```python
from build123d import *

# Parameters (mm, degrees)
F0_W      = 551
F0_H      = 330
F0_W_2    = 543
F0_H_2    = 320
F1_DEPTH  = 180
F3_DEPTH  = 551.001
F4_W      = 10
F4_H      = 30
F5_DEPTH  = 551
F6_W      = 5
F6_H      = 30
F7_DEPTH  = 160
F8_W      = 5
F8_H      = 30
F9_DEPTH  = 160
F10_R     = 10
F11_DEPTH = 25
F12_DEPTH = 170.001
F13_R     = 10
F14_DEPTH = 25


with BuildPart() as f1:
    # F0 (on Front) → F1 (new body)
    with BuildSketch(Plane.XZ):
        with Locations((275.5, 165)):
            Rectangle(F0_W, F0_H)
        with Locations((275.5, 165)):
            Rectangle(F0_W_2, F0_H_2, mode=Mode.SUBTRACT)
    extrude(amount=F1_DEPTH)

    # F2 (on face) → F3 (cut, through all)
    with BuildSketch(Plane.YZ.offset(551)):
        with BuildLine():
            Line((-180, 120), (-180, 210))
            ThreePointArc((-180, 210), (-225, 165), (-180, 120))
        make_face()
        with BuildLine():
            ThreePointArc((-180, 120), (-148.180195, 133.180195), (-135, 165))
            ThreePointArc((-135, 165), (-148.180195, 196.819805), (-180, 210))
            Line((-180, 210), (-180, 120))
        make_face()
    extrude(amount=-F3_DEPTH, mode=Mode.SUBTRACT)

    # F4 (on face) → F5 (join, through all)
    with BuildSketch(Plane.YZ.offset(551)):
        with Locations((-175, -15)):
            Rectangle(F4_W, F4_H)
        with Locations((-5, -15)):
            Rectangle(F4_W, F4_H)
        with Locations((-175, 345)):
            Rectangle(F4_W, F4_H)
        with Locations((-5, 345)):
            Rectangle(F4_W, F4_H)
    extrude(amount=-F5_DEPTH)

    # F6 (on face) → F7 (join, through all)
    with BuildSketch(Plane.XZ.offset(10)):
        with Locations((110.6, -15)):
            Rectangle(F6_W, F6_H)
        with Locations((221.2, -15)):
            Rectangle(F6_W, F6_H)
        with Locations((331.8, -15)):
            Rectangle(F6_W, F6_H)
        with Locations((442.4, -15)):
            Rectangle(F6_W, F6_H)
    extrude(amount=F7_DEPTH)

    # F8 (on face) → F9 (join, through all)
    with BuildSketch(Plane.XZ.offset(10)):
        with Locations((440.4, 345)):
            Rectangle(F8_W, F8_H)
        with Locations((329.8, 345)):
            Rectangle(F8_W, F8_H)
        with Locations((219.2, 345)):
            Rectangle(F8_W, F8_H)
        with Locations((108.6, 345)):
            Rectangle(F8_W, F8_H)
    extrude(amount=F9_DEPTH)

    # F10 (on face) → F11 (cut)
    with BuildSketch(Plane(origin=(0, -170, 0), x_dir=(-1, 0, 0), z_dir=(0, 1, 0))):
        with Locations((-165.959219, -12.5)):
            Circle(F10_R)
        with Locations((-387.1, -12.5)):
            Circle(F10_R)
        with Locations((-163.9, 345)):
            Circle(F10_R)
        with Locations((-385.1, 342.5)):
            Circle(F10_R)
    extrude(amount=-F11_DEPTH, mode=Mode.SUBTRACT)

    # F10 (on face) → F12 (cut, through all)
    with BuildSketch(Plane(origin=(0, -170, 0), x_dir=(-1, 0, 0), z_dir=(0, 1, 0))):
        with Locations((-163.9, 345)):
            Circle(F10_R)
        with Locations((-385.1, 342.5)):
            Circle(F10_R)
        with Locations((-165.959219, -12.5)):
            Circle(F10_R)
        with Locations((-387.1, -12.5)):
            Circle(F10_R)
    extrude(amount=F12_DEPTH, mode=Mode.SUBTRACT)

    # F13 (on face) → F14 (cut)
    with BuildSketch(Plane.XZ.offset(180)):
        with Locations((274.5, 342.5)):
            Circle(F13_R)
        with Locations((276.5, -12.5)):
            Circle(F13_R)
    extrude(amount=-F14_DEPTH, mode=Mode.SUBTRACT)


solid = f1.part
```
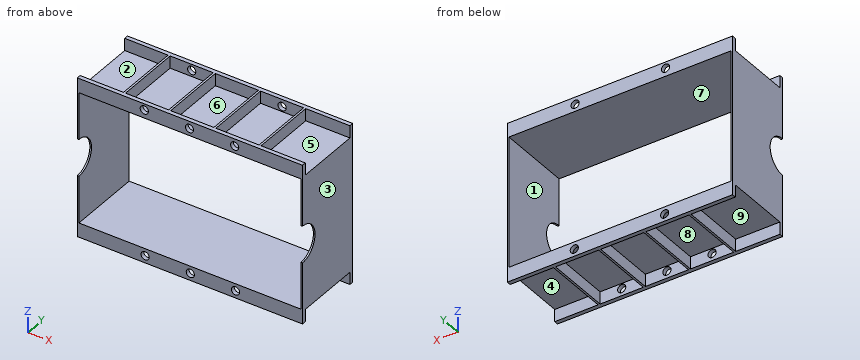
CAD build for the part. Positions are in the model's coordinates, mm. Face numbers are marked on the shaded views. A direction names the side the tool comes from. Coordinates: 2 decimals unless noted, no trailing zeros. Write each loop counter-clockwise with the first axis right and the second up, starting at its lowest first coordinate (ties: lowest second). Pieces come first, ordered by that corner, then holes. Notation, with made-up numbers: (-4.5, 57) -> (32.5, 57) arc R29 cw to (32.5, 92) -> close; hole circle Ø8 at (34.5, 81). An arc over 180 degrees is marked (long way). Return JSON: item names as keys, results as strings. Group by question number.
Q1. Pull direction Z, two halves, no side cores. Call the marked faces 1, 2, 3 and 4: released by +Z, released by -Z, zero draft, split by the parting line, or undercut.
Q2. Flat gauge pins, fed straight in: pin 1 (10 mm diameter, centred on x = 170.5, y = -144, fed in from -Z); pin 2 (3 mm diameter, centred on y = -66.5, z = 288, fed in from -X); pin 3 (2 mm diameter, centred on x = 163.5, y = -130, fed in from +Z); pin 4 (9 mm diameter, centred on y = -76.5, z = -9, fed in from -X). Where does each tip first touch, or does it go through?
Q3. Which spindle directions (+Z, -Z, +X, -X, +Y, -Y) get a long thin tool onto all of the face, cutting with end or side? Do the marked faces 5, 6, 7, 8 and 9. Say none if no direction does.
Q4. Drill centre lines: line 1 (X direction, y = -7.5, z = -12.5); line 2 (Z direction, x = 276, y = -176); line 3 (Z direction, x = 521, y = -143). Where is each one in solid material? Low to high.
Q5. Cut at C-C, the plane x = 163.9. State how many separate pieces and enclosed holes the cut face has, then the cut area to 3 significant figures.
Q6. Cut at B-B, the plane z = 232.5. Give the cut face in (x, y).
Q7. Cut at A-A, the plane x = 301.5. Give the cut face in (y, z), then the cut area to 3 significant figures.
Returned:
{
 "1": {"face 1": "undercut", "face 2": "released by +Z", "face 3": "zero draft", "face 4": "released by -Z"},
 "2": {"pin 1": "stops at z = 0", "pin 2": "stops at x = 0", "pin 3": "stops at z = 330", "pin 4": "stops at x = 108.1"},
 "3": {"face 5": "+Z, +X", "face 6": "+Z", "face 7": "+Y, -Y", "face 8": "-Z", "face 9": "-Z, -X"},
 "4": {"line 1": "x = 0 to 155.96, 175.96 to 377.1, 397.1 to 551", "line 2": "z = -30 to -22.49, -2.51 to 5, 325 to 332.61, 352.39 to 360", "line 3": "z = 0 to 5, 325 to 330"},
 "5": {"separate pieces": "6", "enclosed holes": "0", "area": "2,210 mm2"},
 "6": {"outline": "(0, -180) -> (4, -180) -> (4, 0) -> (0, 0) -> close; (547, -180) -> (551, -180) -> (551, 0) -> (547, 0) -> close"},
 "7": {"outline": "(-180, -30) -> (-170, -30) -> (-170, 0) -> (-10, 0) -> (-10, -30) -> (0, -30) -> (0, 5) -> (-180, 5) -> close; (-180, 325) -> (0, 325) -> (0, 360) -> (-10, 360) -> (-10, 330) -> (-170, 330) -> (-170, 360) -> (-180, 360) -> close", "area": "3,000 mm2"}
}
